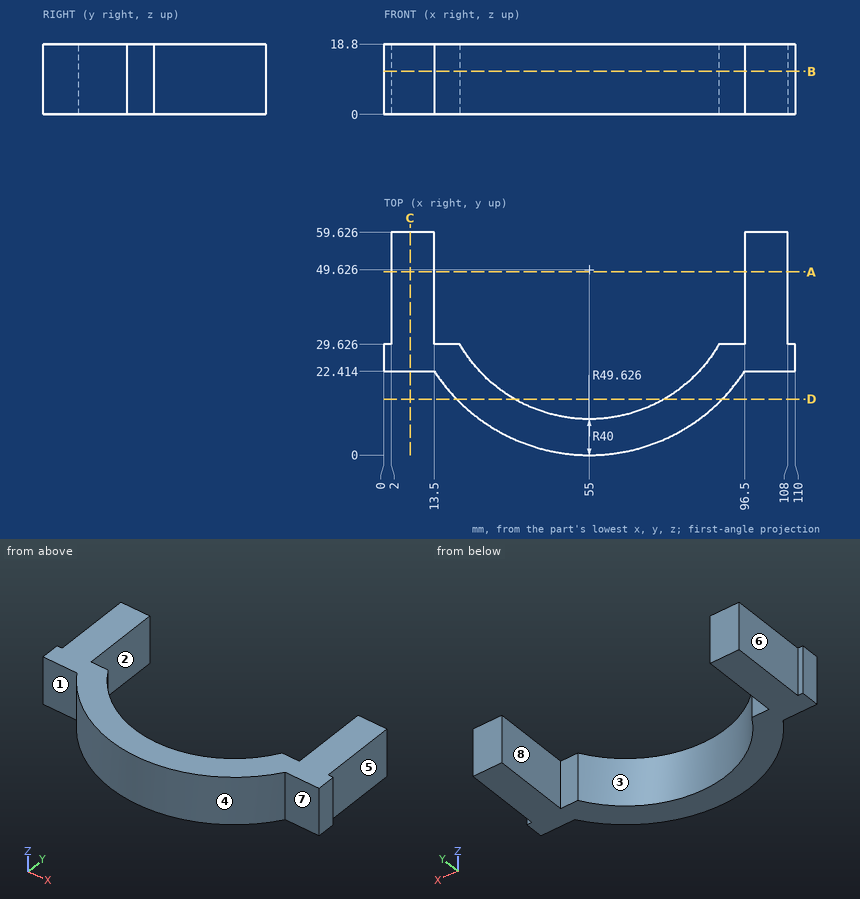
Design review of the part shown in the three views and the two pictorial views. Dimensions are in mm from the part's minimum x, y and z. A direction names the side the tool comes from. Give positions to 0.01 mm unless a question says otherwise; leave off trailing zeros. Write each loop counter-clockwise with the first axis right and the second up, starting at its lowest first coordinate (ties: lowest second). Pieces come first, ordered by that corner, then holes.
(1) Wall thickness on line 1 along X through (y, z) = (54.5, 17.75); line 2 along X through (y, z) = (22, 11.25) (1 decimal); line 3 along Y through (x, z) = (102, 17): over which ranges is each line inside the solid? List them lowest first.
Checked values:
line 1: x = 2 to 13.5, 96.5 to 108
line 2: x = 13.8 to 26.1, 83.9 to 96.2
line 3: y = 22.41 to 59.63
(2) Clearance check with flat-ended pins moving along their axes: pin 1 Ø8 at (y, z) = (8.5, 10) entering from +X; pin 2 Ø3.5 at (x, z) = (16.5, 5.5) entering from +Y; pin 3 Ø2 at (x, z) = (15, 15) entering from -Y. State where each tip first meets the part, or that it passes through.
Checked values:
pin 1: stops at x = 87.93
pin 2: stops at y = 29.63
pin 3: stops at y = 18.94
(3) Add section C-C (x = 7). Give the boundary of the cut face in (y, z), and give its area (3 significant figures).
Checked values:
outline: (22.41, 0) - (59.63, 0) - (59.63, 18.8) - (22.41, 18.8) - close
area: 700 mm2
(4) Add section B-B (z = 11.5). Give the boundary of the cut face in (x, y), and give its area (3 significant figures).
Checked values:
outline: (0, 22.41) - (13.5, 22.41) arc R49.63 ccw to (96.5, 22.41) - (110, 22.41) - (110, 29.63) - (108, 29.63) - (108, 59.63) - (96.5, 59.63) - (96.5, 29.63) - (89.64, 29.63) arc R40 cw to (20.36, 29.63) - (13.5, 29.63) - (13.5, 59.63) - (2, 59.63) - (2, 29.63) - (0, 29.63) - close
area: 1,810 mm2
(5) Add section A-A (y = 49). Give the boundary of the cut face in (x, z).
Checked values:
outline: (2, 0) - (13.5, 0) - (13.5, 18.8) - (2, 18.8) - close; (96.5, 0) - (108, 0) - (108, 18.8) - (96.5, 18.8) - close
(6) Tool access review of the marked faces 5, 6, 7 and 8: name each direction out of +Z, -Z, +X, -X, +Y, -Y from which nothing blocks a thin tool from reaching the whole face with its end or side.
Checked values:
face 5: +Z, -Z, +X, +Y
face 6: +Z, -Z, -X, +Y
face 7: +Z, -Z, +X, -Y
face 8: +Z, -Z, +Y
(7) Add section D-D (y = 15). Give the boundary of the cut face in (x, z), and give its area (3 significant figures).
Checked values:
outline: (19.45, 0) - (34.97, 0) - (34.97, 18.8) - (19.45, 18.8) - close; (75.03, 0) - (90.55, 0) - (90.55, 18.8) - (75.03, 18.8) - close
area: 584 mm2
(8) Mouldability with a two-part tool opening along X and no side actions: class the marked faces 1, 2, 3 and 4 as +X half, -X half, draft (parallel to the pull), parting line (faces both ways), or undercut.
Checked values:
face 1: draft
face 2: undercut
face 3: undercut
face 4: parting line
